Could you check a few things on this model? Use its own coordinates, in mm. A direction names the side the tool comes from. Round coordinates to 2 decimals unless told otherwise and drop trailing zeros. Order: outer loops, then holes, each group sorted by start corner. A loop starts at its lowest first (then second) coordinate and runs counter-clockwise, first axis right, second up.
```python
from build123d import *

# Parameters (mm, degrees)
SKETCH1_W           = 26.4
SKETCH1_H           = 1.4
BOSS_EXTRUDE1_DEPTH = 30
BOSS_EXTRUDE2_DEPTH = 3


with BuildPart() as part:
    # Sketch1 → Boss-Extrude1 (new body)
    with BuildSketch(Plane.XY):
        with Locations((13.2, 0.7)):
            Rectangle(SKETCH1_W, SKETCH1_H)
    extrude(amount=BOSS_EXTRUDE1_DEPTH)

    # Sketch2 → Boss-Extrude2 (add)
    with BuildSketch(Plane.XY.offset(30)):
        Polygon((4.2, 1.4), (4.2, 2.4), (5.2, 3.4), (21.2, 3.4), (22.2, 2.4), (22.2, 1.4), align=None)
    extrude(amount=-BOSS_EXTRUDE2_DEPTH)


solid = part.part
```
Q1. Imagine slicing it at C-C, the plane x = 2.5. Please give me the cut outline in (y, z).
Q2. Imagine slicing it at A-A, the plane z = 28.25. Please give me the cut outline in (x, y).
Q3. For faces 1 (the flat face through (22.2, 2, 29)), 2 (the flat face through (4.2, 2, 29)), 3 (the flat face through (26.4, 1, 15)), 4 (the flat face through (13, 2, 27)), which set-ups out of +Z, -Z, +X, -X, +Y, -Y let a thin tool reach every point of the face, with its end or its side?
Q4. Imagine slicing it at D-D, the plane z = 11.25. Please give me the cut outline in (x, y).
Q5. For P1, Ø1, axis at x = 11, y = 2.5, coming from the -Z side; P2, Ø0.8, axis at y = 2, z = 29, coming from the -X side; P3, Ø4, axis at x = 3, z = 5.5, coming from the +Y side, each with a flat end and sliding along its axis, tell me the tip position at first contact or that it passes through.
Q6. I need wall thicknesses on L1, parallel to Y at x = 15.75, z = 5; L2, parallel to Z at x = 19.75, y = 2.35. Which ranges of each line are inside material? Lowest first, please.
Q7. Imagine slicing it at B-B, the plane x = 10.25. Please give me the cut outline in (y, z).
Filled in:
1. outline: (0, 0) - (1.4, 0) - (1.4, 30) - (0, 30) - close
2. outline: (0, 0) - (26.4, 0) - (26.4, 1.4) - (22.2, 1.4) - (22.2, 2.4) - (21.2, 3.4) - (5.2, 3.4) - (4.2, 2.4) - (4.2, 1.4) - (0, 1.4) - close
3. face 1: +Z, -Z, +X, +Y
3. face 2: +Z, -Z, -X, +Y
3. face 3: +Z, -Z, +X, +Y, -Y
3. face 4: -Z, +X, -X, +Y
4. outline: (0, 0) - (26.4, 0) - (26.4, 1.4) - (0, 1.4) - close
5. P1: stops at z = 27
5. P2: stops at x = 4.2
5. P3: stops at y = 1.4
6. L1: y = 0 to 1.4
6. L2: z = 27 to 30
7. outline: (0, 0) - (1.4, 0) - (1.4, 27) - (3.4, 27) - (3.4, 30) - (0, 30) - close
